For this review, take the finished solid that the model builds, in its own axes (mm). Round coordinates to 2 decimals unless told otherwise and drop trailing zeros. Write each loop counter-clockwise with the first axis right and the second up, starting at its lowest first coordinate (ties: lowest second). Pieces come first, ordered by that corner, then holes. Notation, with made-up numbers: (-14, -37.75) -> (-5, -37.75) arc R16 ccw to (-5, -12.75) -> close; hole circle Ø4 at (9.5, -15.5). An arc over 180 degrees is marked (long way). Write item = value, one per line. Start each with the question number.
Autodesk Inventor part; units mm, degrees
ref_plane "YZ Plane" through (0, 0, 0) normal (1, 0, 0) x (0, 1, 0)
ref_plane "XZ Plane" through (0, 0, 0) normal (0, 1, 0) x (-1, 0, 0)
ref_plane "XY Plane" through (0, 0, 0) normal (0, 0, 1) x (1, 0, 0)
sketch "Sketch1" plane through (0, 0, 0) normal (0, 0, 1) x (1, 0, 0)
  line L0 (-475, -300) -> (475, -300)
  line L1 (475, -300) -> (475, 300)
  line L2 (475, 300) -> (-475, 300)
  line L3 (-475, 300) -> (-475, -300)
  line L4 (-475, -300) -> (475, 300) construction
  line L5 (475, -300) -> (-475, 300) construction
  point P0 (0, 0)
  dimension "d0" = 950
  dimension "d1" = 600
extrude "Plate1" add sketch "Sketch1" along normal blind 5
fillet "Corner Round1" radius 15 4 edges at (475, 300, 2.5) (475, -300, 2.5) (-475, -300, 2.5) (-475, 300, 2.5)
sketch "Sketch2" plane through (0, 0, 5) normal (0, 0, 1) x (1, 0, 0)
  line L0 (-475, 300) -> (-475, -300)
  line L1 (-475, 0) -> (475, 0)
  line L2 (475, -300) -> (475, 300)
  line L3 (475, 300) -> (-475, 300)
  line L4 (0, 300) -> (0, -300)
  line L5 (475, -300) -> (-475, -300)
  line L6 (-200, 295) -> (200, 295)
  line L7 (200, 295) -> (200, 289.92)
  line L8 (200, 289.92) -> (-200, 289.92)
  line L9 (-200, 289.92) -> (-200, 295)
  line L10 (-200, 295) -> (200, 289.92) construction
  line L11 (200, 295) -> (-200, 289.92) construction
  line L12 (-475, 300) -> (475, 300)
  line L13 (-470, -100) -> (-464.92, -100)
  line L14 (-464.92, -100) -> (-464.92, 100)
  line L15 (-464.92, 100) -> (-470, 100)
  line L16 (-470, 100) -> (-470, -100)
  line L17 (-470, -100) -> (-464.92, 100) construction
  line L18 (-464.92, -100) -> (-470, 100) construction
  line L19 (-475, -300) -> (-475, 300)
  line L20 (-200, -289.92) -> (-200, -295)
  line L21 (-200, -295) -> (200, -295)
  line L22 (200, -295) -> (200, -289.92)
  line L23 (-200, -295) -> (200, -289.92) construction
  line L24 (200, -295) -> (-200, -289.92) construction
  line L25 (200, -289.92) -> (-200, -289.92)
  line L26 (464.92, 100) -> (470, 100)
  line L27 (464.92, -100) -> (464.92, 100)
  line L28 (470, -100) -> (464.92, 100) construction
  line L29 (470, -100) -> (464.92, -100)
  line L30 (464.92, -100) -> (470, 100) construction
  line L31 (470, 100) -> (470, -100)
  point P0 (0, 0)
  point P1 (44.3571, 22.9179)
  point P2 (0, 292.46)
  point P3 (0, 295)
  point P4 (-467.46, 0)
  point P5 (-470, 0)
  point P6 (0, -292.46)
  point P7 (0, -295)
  point P8 (0, -300)
  point P9 (0, -300)
  point P10 (467.46, 0)
  point P11 (470, 0)
  point P12 (0, 0)
  dimension "d4" = 5.08
  dimension "d5" = 400
  dimension "d6" = 5
  dimension "d7" = 5.08
  dimension "d8" = 200
  dimension "d9" = 5
  dimension "d10" = 950
  dimension "d11" = 600
extrude "Cut1" cut sketch "Sketch2" against normal blind 5 contours L16 L15 L14 L1 | L1 L14 L13 L16 | L6 L7 L8 L4 | L4 L8 L9 L6 | L21 L20 L25 L4 | L4 L25 L22 L21 | L31 L29 L27 L1 | L1 L27 L26 L31
equation "\"d14\" = Thickness"
equation "\"d2\" = Thickness"
equation "\"BendRadius\" = Thickness"
equation "\"BendReliefWidth\" = Thickness"
equation "\"BendReliefDepth\" = 0.5 * Thickness"
equation "\"TransitionRadius\" = BendRadius"
equation "\"JacobiRadiusSize\" = BendRadius"
equation "\"GapSize\" = Thickness"
properties part number "Base Full Game"
1. Wall thickness on L1, parallel to X at y = 47, z = 0.85; L2, parallel to Y at x = 166, z = 3.4: over which ranges is each line inside the solid? List them lowest first. Write a range as from..to.
2. Clearance check with flat-ended pins moving along their axes: pin 1 Ø1.5 at (x, z) = (-467.5, 2) entering from -Y; pin 2 Ø2.5 at (x, z) = (467, 1.5) entering from +Y. State where each tip first meets the part, or that it passes through.
3. Consider section A-A, the plane x = -27. Give the boundary of the cut face in (y, z).
Outcome:
q1.L1 = -475..-470, -464.92..464.92, 470..475
q1.L2 = -300..-295, -289.92..289.92, 295..300
q2.pin_1 = -298.4
q2.pin_2 = 298.85
q3.outline = (-300, 0) -> (-295, 0) -> (-295, 5) -> (-300, 5) -> close; (-289.92, 0) -> (289.92, 0) -> (289.92, 5) -> (-289.92, 5) -> close; (295, 0) -> (300, 0) -> (300, 5) -> (295, 5) -> close
